Build history of the part. All positions in model axes, mm. Face numbers are marked on the shaded views. A direction names the side the tool comes from. Give positions to 0.01 mm unless a question says otherwise; leave off trailing zeros. Answer as a JSON object with one key per item and string values. Group by question number.
Q1. Two-plate mould, pull along X, no slides. Class the marked faces 1 and 2: pulls with the +X half, pulls with the -X half, needs draft (parallel to the pull), parting line crosses it, or undercut.
Q2. Drop flat-ended pins along their axis: pin 1 (2 mm diameter, centred on y = 0, z = -0.5, fed in from +X); pin 2 (7 mm diameter, centred on x = 2, y = 0, fed in from -Z); pin 3 (1 mm diameter, centred on y = -5, z = -1, fed in from -X). Give the stop position or say it passes through.
Q3. Band-saw the part on A-A, the plane y = 17. Count the separate pieces of the cut face and the enclosed holes in it, plus the area to 3 significant figures.
Q4. Wall check: probe 1 along Y at (x, z) = (18, 2.25); probe 2 along X at (y, z) = (14, 1.5); probe 3 along Y at (x, z) = (0, 0.8). Give the ranges that are in metal, low to high. Write a range as from..to.
Q5. Tool access for the marked faces 3, 4 and 5: list every direction of +Z, -Z, +X, -X, +Y, -Y with a clear straight run to the whole face (end or side of a thin tool).
Autodesk Inventor part; units mm, degrees
ref_plane "YZ Plane" through (0, 0, 0) normal (1, 0, 0) x (0, 1, 0)
ref_plane "XZ Plane" through (0, 0, 0) normal (0, 1, 0) x (-1, 0, 0)
ref_plane "XY Plane" through (0, 0, 0) normal (0, 0, 1) x (1, 0, 0)
sketch "Sketch1" plane through (0, 0, 0) normal (0, 0, 1) x (1, 0, 0)
  circle A0 centre (0, 0) radius 36.9824
  dimension "d17" = 73.9648
extrude "Extrusion1" add sketch "Sketch1" along normal mid plane 6.35
sketch "Sketch4" plane through (0, 0, 0) normal (1, 0, 0) x (0, 1, 0)
  circle A0 centre (36.9824, 0) radius 1.7653
  line L0 (36.9824, -3.175) -> (36.9824, 3.175) construction
  line L1 (36.9824, -3.175) -> (36.9824, 3.175)
  line L2 (36.9824, -3.175) -> (36.9824, 3.175)
  line L3 (0, -6.8515) -> (0, 6.9022)
  point P0 (0, 0)
  dimension "d5" = 3.5306
revolve "Revolution1" cut sketch "Sketch4" angle 360 about axis through (0, 0, -6.8515) along (0, 0, 1)
sketch "Sketch5" plane through (0, -10.4797, 3.175) normal (0, 0, 1) x (1, 0, 0)
  line L0 (11.3113, 29.5816) -> (18.1134, 29.6722)
  line L1 (18.1134, 29.6722) -> (21.5928, 23.8267)
  line L2 (21.5928, 23.8267) -> (18.2702, 17.8907)
  line L3 (18.2702, 17.8907) -> (11.4682, 17.8001)
  line L4 (11.4682, 17.8001) -> (7.9887, 23.6456)
  line L5 (7.9887, 23.6456) -> (11.3113, 29.5816)
  line L6 (-18.0537, 29.5853) -> (-11.2517, 29.6759)
  line L7 (-11.2517, 29.6759) -> (-7.7722, 23.8304)
  line L8 (-7.7722, 23.8304) -> (-11.0948, 17.8944)
  line L9 (-11.0948, 17.8944) -> (-17.8969, 17.8038)
  line L10 (-17.8969, 17.8038) -> (-21.3763, 23.6493)
  line L11 (-21.3763, 23.6493) -> (-18.0537, 29.5853)
  line L12 (-17.916, 3.9729) -> (-11.114, 4.0635)
  line L13 (-11.114, 4.0635) -> (-7.6345, -1.782)
  line L14 (-7.6345, -1.782) -> (-10.9571, -7.718)
  line L15 (-10.9571, -7.718) -> (-17.7592, -7.8086)
  line L16 (-17.7592, -7.8086) -> (-21.2386, -1.9631)
  line L17 (-21.2386, -1.9631) -> (-17.916, 3.9729)
  line L18 (11.6578, 3.5557) -> (18.4598, 3.6463)
  line L19 (18.4598, 3.6463) -> (21.9393, -2.1992)
  line L20 (21.9393, -2.1992) -> (18.6167, -8.1352)
  line L21 (18.6167, -8.1352) -> (11.8146, -8.2257)
  line L22 (11.8146, -8.2257) -> (8.3352, -2.3803)
  line L23 (8.3352, -2.3803) -> (11.6578, 3.5557)
  line L24 (-23.7615, 10.4722) -> (-31.2466, 6.34)
  line L25 (-31.2466, 6.34) -> (-31.0827, 14.8884)
  line L26 (-31.0827, 14.8884) -> (-23.7615, 10.4722)
  line L27 (23.8373, 10.4722) -> (31.6292, 14.9709)
  line L28 (31.6292, 14.9709) -> (31.6292, 5.9736)
  line L29 (31.6292, 5.9736) -> (23.8373, 10.4722)
  line L30 (2.3663, 35.8446) -> (-2.7917, 35.9364)
  line L31 (-2.7917, 35.9364) -> (-0.1332, 40.3574)
  line L32 (-0.1332, 40.3574) -> (2.3663, 35.8446)
  line L33 (2.3663, -13.8498) -> (-0.0945, -18.246)
  line L34 (-0.0945, -18.246) -> (-2.6714, -13.9168)
  line L35 (-2.6714, -13.9168) -> (2.3663, -13.8498)
  point P0 (0, 10.4797)
  point P1 (14.7908, 23.7362)
  point P2 (-14.5743, 23.7399)
  point P3 (-14.4366, -1.8725)
  point P4 (15.1372, -2.2897)
  point P5 (-28.6969, 10.5669)
  point P6 (29.0319, 10.4722)
  point P7 (-0.1862, 37.3795)
  point P8 (-0.1332, -15.3375)
extrude "Extrusion3" cut sketch "Sketch5" against normal through all
sketch "Sketch6" plane through (0, -10.4797, 3.175) normal (0, 0, 1) x (1, 0, 0)
  circle A0 centre (0, 10.4797) radius 1.524
  circle A1 centre (0, 10.4797) radius 36.9824
  dimension "d9" = 3.048
extrude "Extrusion4" cut sketch "Sketch6" against normal through all contours A0
sketch "Sketch9" plane through (0, 0, -3.175) normal (0, 0, -1) x (-1, 0, 0)
  circle A0 centre (0, 0) radius 4.445
  circle A1 centre (0, 0) radius 1.524
  dimension "d14" = 8.89
extrude "Extrusion5" cut sketch "Sketch9" against normal blind 3.175
sketch "Sketch11" plane through (0, -10.4797, -3.175) normal (0, 0, -1) x (-1, 0, 0)
  arc A0 (6.84, 6.338) -> (19.5394, 8.1514) centre (2.6508, 81.0506) ccw
  arc A1 (19.5394, 8.1514) -> (19.5394, 12.8081) centre (19, 10.4797) ccw
  arc A2 (19.5394, 12.8081) -> (6.84, 14.6214) centre (2.6508, -60.0911) ccw
  arc A3 (4.1417, 17.3197) -> (2.3283, 30.0191) centre (-70.5709, 13.1305) ccw
  arc A4 (2.3283, 30.0191) -> (-2.3283, 30.0191) centre (0, 29.4797) ccw
  arc A5 (-2.3283, 30.0191) -> (-4.1417, 17.3197) centre (70.5709, 13.1305) ccw
  arc A6 (-6.84, 14.6214) -> (-19.5394, 12.8081) centre (-2.6508, -60.0911) ccw
  arc A7 (-19.5394, 12.8081) -> (-19.5394, 8.1514) centre (-19, 10.4797) ccw
  arc A8 (-19.5394, 8.1514) -> (-6.84, 6.338) centre (-2.6508, 81.0506) ccw
  arc A9 (-4.1417, 3.6397) -> (-2.3283, -9.0597) centre (70.5709, 7.8289) ccw
  arc A10 (-2.3283, -9.0597) -> (2.3283, -9.0597) centre (0, -8.5203) ccw
  arc A11 (2.3283, -9.0597) -> (4.1417, 3.6397) centre (-70.5709, 7.8289) ccw
  circle A12 centre (0, 20.7297) radius 0.4953
  circle A13 centre (0, 23.7197) radius 0.4953
  circle A14 centre (0, 26.4497) radius 0.4953
  circle A15 centre (0, 17.8197) radius 0.5
  circle A16 centre (0, 10.4797) radius 2.9464
  circle A17 centre (-7.34, 10.4797) radius 0.5
  circle A18 centre (-10.25, 10.4797) radius 0.4953
  circle A19 centre (-13.24, 10.4797) radius 0.4953
  circle A20 centre (-15.97, 10.4797) radius 0.4953
  circle A21 centre (7.34, 10.4797) radius 0.5
  circle A22 centre (10.25, 10.4797) radius 0.4953
  circle A23 centre (13.24, 10.4797) radius 0.4953
  circle A24 centre (15.97, 10.4797) radius 0.4953
  circle A25 centre (0, 3.1397) radius 0.5
  circle A26 centre (0, 0.2297) radius 0.4953
  circle A27 centre (0, -2.7603) radius 0.4953
  circle A28 centre (0, -5.4903) radius 0.4953
  line L0 (-4.1417, 17.3197) -> (-6.84, 14.6214)
  line L1 (4.1417, 17.3197) -> (6.84, 14.6214)
  line L2 (6.84, 6.338) -> (4.1417, 3.6397)
  line L3 (-6.84, 6.338) -> (-4.1417, 3.6397)
extrude "Extrusion6" cut sketch "Sketch11" against normal blind 2.032 contours L2 A11 A10 A9 L3 A8 A7 A6 L0 A5 A4 A3 L1 A2 A1 A0 | A12 | A13 | A14 | A15 | A17 | A18 | A19 | A20 | A21 | A22 | A23 | A24 | A25 | A26 | A27 | A28
sketch "Sketch12" plane through (0, 0, 3.175) normal (0, 0, 1) x (1, 0, 0)
  circle A0 centre (0, 0) radius 1.778
  dimension "d20" = 3.556
extrude "Extrusion7" cut sketch "Sketch12" against normal blind 1.27
properties part number "Hew O Ring"
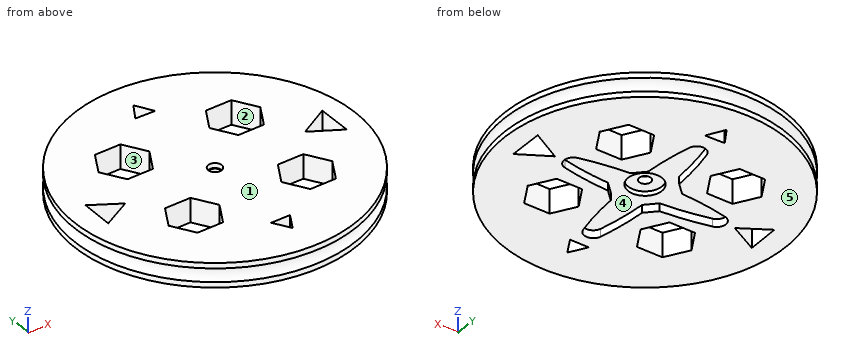
Worked answers:
{
 "1": {"face 1": "needs draft", "face 2": "undercut"},
 "2": {"pin 1": "x = 36.05", "pin 2": "z = -1.14", "pin 3": "x = -35.71"},
 "3": {"separate pieces": "3", "enclosed holes": "0", "area": "276 mm2"},
 "4": {"probe 1": "-32.31..-18.62, -6.84..7.41, 19.19..32.31", "probe 2": "-33.22..-20.91, -8.16..8.46, 21.2..33.22", "probe 3": "-35.41..-28.56, -24.36..-1.52, 1.52..25.41, 29.64..35.41"},
 "5": {"face 3": "+Z, -Z", "face 4": "-Z", "face 5": "-Z, +X, -X, +Y, -Y"}
}
